Job drawing, mm, ordinate dimensions from the low corner. One solid piece. Round coordinates to 2 decimals unless told otherwise and drop trailing zeros. Write each loop counter-clockwise with the first axis right and the second up, starting at its lowest first coordinate (ties: lowest second). Pieces come first, ordered by that corner, then holes.
1) Saw through at B-B on z = 97.5. Write the cut outline in (x, y), and give its area (3 significant figures).
2) Saw through at D-D on y = 3.9. Count the separate pieces of the cut face and the enclosed holes in it, and give its area (3 significant figures).
3) Drill centre lines: L1, parallel to Z at x = 22, y = 4.45; L2, parallel to Z at x = 122.5, y = 3.55 (1 decimal); L3, parallel to X at y = 3.7, z = 71. Where is each one in solid material? Low to high.
4) Saw through at C-C on x = 73. Write the cut outline in (y, z).
5) Flat gauge pins, fed straight in: pin 1 (10 mm diameter, centred on x = 152.15, z = 130.78, fed in from -Y); pin 2 (1.4 mm diameter, centred on x = 189, y = 3, fed in from +Z). Where does each tip first touch, or does it go through?
6) Saw through at A-A on x = 101.6. Write the cut outline in (y, z).
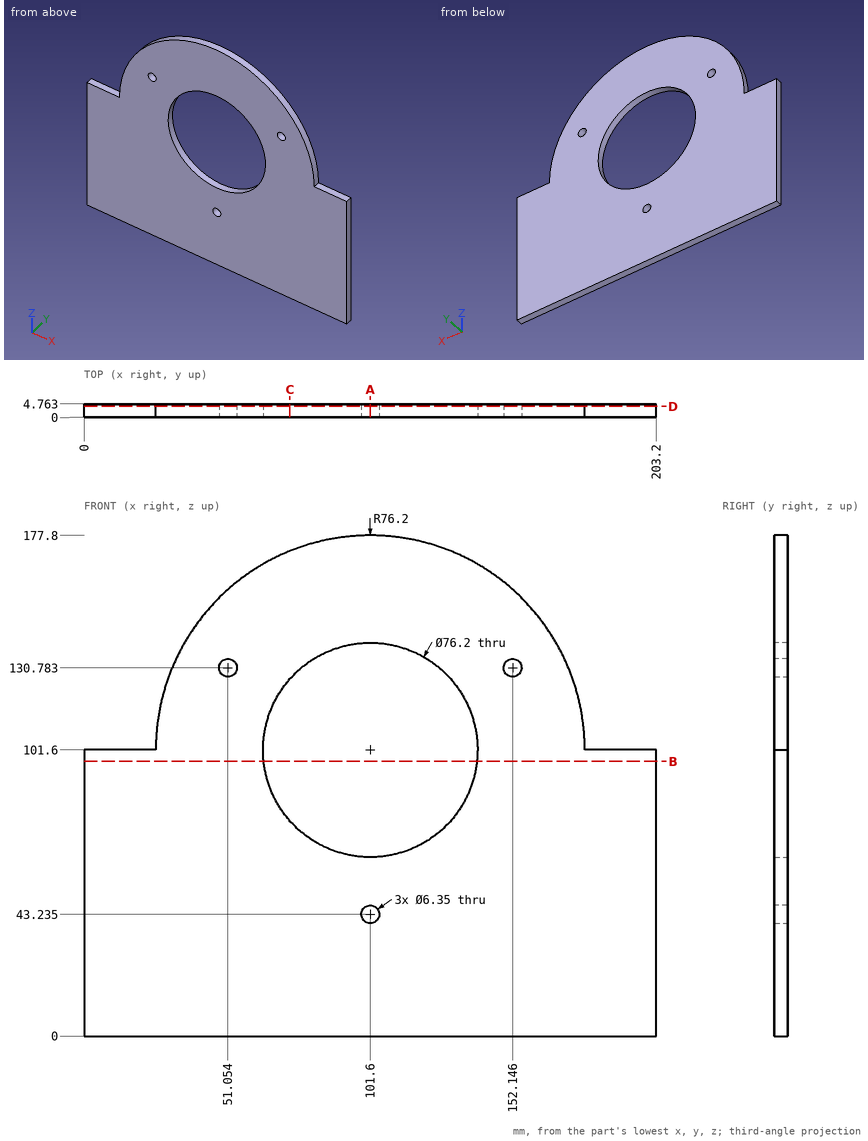
Completed:
1. outline: (0, 0) - (63.72, 0) - (63.72, 4.76) - (0, 4.76) - close; (139.48, 0) - (203.2, 0) - (203.2, 4.76) - (139.48, 4.76) - close
1. area: 607 mm2
2. separate pieces: 1
2. enclosed holes: 4
2. area: 25,100 mm2
3. L1: z = 0 to 101.6
3. L2: z = 0 to 69.7, 133.5 to 174.9
3. L3: x = 0 to 78.9, 124.3 to 203.2
4. outline: (0, 0) - (4.76, 0) - (4.76, 76.43) - (0, 76.43) - close; (0, 126.77) - (4.76, 126.77) - (4.76, 172.23) - (0, 172.23) - close
5. pin 1: stops at y = 0
5. pin 2: stops at z = 101.6
6. outline: (0, 0) - (4.76, 0) - (4.76, 40.06) - (0, 40.06) - close; (0, 46.41) - (4.76, 46.41) - (4.76, 63.5) - (0, 63.5) - close; (0, 139.7) - (4.76, 139.7) - (4.76, 177.8) - (0, 177.8) - close
